from build123d import *


with BuildPart() as part:
    # Skizze1 → Welle (revolve)
    with BuildSketch(Plane.XY, mode=Mode.PRIVATE) as welle_sk:
        Polygon((0, 0), (0, 9), (1, 10), (20, 10), (20, 12.5), (40, 12.5), (40, 16), (120, 16), (120, 12.5), (140, 12.5), (140, 8), (159, 8), (160, 7), (160, 0), align=None)
    revolve(welle_sk.sketch.rotate(Axis((-5, 0, 0), (1, 0, 0)), 90), axis=Axis((-5, 0, 0), (1, 0, 0)))


solid = part.part
Source: CAD feature listing. Evaluate the final solid. Frame: model axes, mm. A direction names the side the tool comes from. Give positions to 0.01 mm unless a question says otherwise; leave off trailing zeros. Write each loop counter-clockwise with the first axis right and the second up, starting at its lowest first coordinate (ties: lowest second). Pieces come first, ordered by that corner, then holes. Notation, with made-up numbers: (36, 50.25) - (92, 50.25) arc R14 ccw to (92, 65.25) - close; hole circle Ø5 at (89.5, -1.5). An arc over 180 degrees is marked (long way). Write item = value, one per line. Start each with the question number.
Q1. Pin query (flat end, axial travel): pin 1 Ø10 at (x, y) = (26, -10.5) entering from +Z (3 decimals); pin 2 Ø12 at (x, y) = (53, 11) entering from -Z; pin 3 Ø6 at (x, y) = (93.5, -3.5) entering from -Z. Return the tip coordinate at first contact, or that it passes through.
Q2. Reachability of faces 1 (the cylindrical face through (80.56, 15.62, -3.47)), 2 (the flat face through (120, 8, -10)), 3 (the flat face through (20, -10.2, 0.1)) from +Z, -Z, +X, -X, +Y, -Y: full face, straight path, thin tool, end or side. Return the list, or none.
Q3. Cut plane C-C, the plane x = 31.5. Return loops of the section in (y, z), then the cut area to 3 significant figures.
Q4. Material intervals for probe 1 along X at (y, z) = (10.5, -8); probe 2 along Y at (x, z) = (103, -12.5); probe 3 along Y at (x, z) = (49, 0), sorted ascending.
Q5. Cut plane D-D, the plane x = 90.5. Return loops of the section in (y, z).
Q6. Cut plane A-A, the plane z = 0. Return loops of the section in (x, y).
Computed values:
q1.pin_1 = 11.225
q1.pin_2 = -15.2
q1.pin_3 = -15.99
q2.face_1 = +X, -X
q2.face_2 = +X
q2.face_3 = -X
q3.outline = circle Ø25 at (0, 0)
q3.area = 491 mm²
q4.probe_1 = 40 to 120
q4.probe_2 = -9.99 to 9.99
q4.probe_3 = -16 to 16
q5.outline = circle Ø32 at (0, 0)
q6.outline = (0, -9) - (1, -10) - (20, -10) - (20, -12.5) - (40, -12.5) - (40, -16) - (120, -16) - (120, -12.5) - (140, -12.5) - (140, -8) - (159, -8) - (160, -7) - (160, 7) - (159, 8) - (140, 8) - (140, 12.5) - (120, 12.5) - (120, 16) - (40, 16) - (40, 12.5) - (20, 12.5) - (20, 10) - (1, 10) - (0, 9) - close
